CAD build for the part. Positions are in the model's coordinates, mm. A direction names the side the tool comes from. Give positions to 0.01 mm unless a question says otherwise; leave off trailing zeros. Loops run counter-clockwise (first coordinate to the right, second up) from the corner with the lowest first, then second, coordinate; pieces in that order, holes last. Notation, with made-up numbers: (-6, -33.5) -> (45, -33.5) arc R21 ccw to (45, -1.5) -> close; hole circle Ø6 at (21, 11). An arc over 180 degrees is marked (long way). Use one line per item in the form item = value.
```python
from build123d import *


with BuildPart() as part:
    # Sketch3 → bearing-revolution (revolve)
    with BuildSketch(Plane.XY):
        with BuildLine():
            Line((0.3048, 3.175), (7.14375, 3.175))
            Line((7.14375, 3.175), (7.14375, 4.445))
            Line((7.14375, 4.445), (5.159375, 4.445))
            Line((5.159375, 4.445), (5.159375, 8.255))
            Line((5.159375, 8.255), (7.14375, 8.255))
            Line((7.14375, 8.255), (7.14375, 9.2202))
            ThreePointArc((7.14375, 9.2202), (7.054476147, 9.435726147), (6.83895, 9.525))
            Line((6.83895, 9.525), (0.3048, 9.525))
            ThreePointArc((0.3048, 9.525), (0.089273853, 9.435726147), (0, 9.2202))
            Line((0, 9.2202), (0, 8.255))
            Line((0, 8.255), (1.984375, 8.255))
            Line((1.984375, 8.255), (1.984375, 4.445))
            Line((1.984375, 4.445), (0, 4.445))
            Line((0, 4.445), (0, 3.4798))
            ThreePointArc((0, 3.4798), (0.089273853, 3.264273853), (0.3048, 3.175))
        make_face()
    revolve(axis=Axis((-4.832058368, 0, 0), (1, 0, 0)))


solid = part.part
```
1. Drill centre lines: line 1 (Z direction, x = 6.5, y = 0) (3 decimals); line 2 (Y direction, x = 6.75, z = -2.75); line 3 (Y direction, x = 1.5, z = -0.75). Where is each one in solid material? Low to high.
Result sheet:
line_1 = -9.525 to -8.255, -4.445 to -3.175, 3.175 to 4.445, 8.255 to 9.525
line_2 = -9.12 to -7.78, -3.49 to -1.59, 1.59 to 3.49, 7.78 to 9.12
line_3 = -9.5 to -8.22, -4.38 to -3.09, 3.09 to 4.38, 8.22 to 9.5
2. Tool access for faces 4 (the cylindrical face through (1.006, 7.874, 2.48)), 5 (the flat face through (7.144, 7, -5)), 6 (the cylindrical face through (6.165, 7.874, 2.48)): list every direction of +Z, -Z, +X, -X, +Y, -Y with a clear straight run to the whole face (end or side of a thin tool).
Result sheet:
face_4 = -X
face_5 = +Z, -Z, +X, +Y, -Y
face_6 = +X
3. Mould opens along Y. For faces 1 (the flat face through (0, 0, -4)), 2 (the cylindrical face through (3.526, -7.559, -5.796)), 3 (the cylindrical face through (6.14, -0.96, -4.34)) say: pulls with the +Y half, pulls with the -Y half, needs draft (parallel to the pull), parting line crosses it, or undercut.
Result sheet:
face_1 = needs draft
face_2 = parting line crosses it
face_3 = undercut
4. Cut at C-C, the plane x = 4.25. Write the cut outline in (y, z) (3 decimals), then the cut area to 3 significant figures.
Result sheet:
outline = circle Ø19.05 at (0, 0); hole circle Ø6.35 at (0, 0)
area = 253 mm^2
5. Drop flat-ended pins along their axis: P1, Ø4, axis at x = 4.5, z = 5, coming from the +Y side; P2, Ø1, axis at y = -5, z = 0, coming from the +X side. Give the stop position or say it passes through.
Result sheet:
P1 = 9.04
P2 = 5.16
